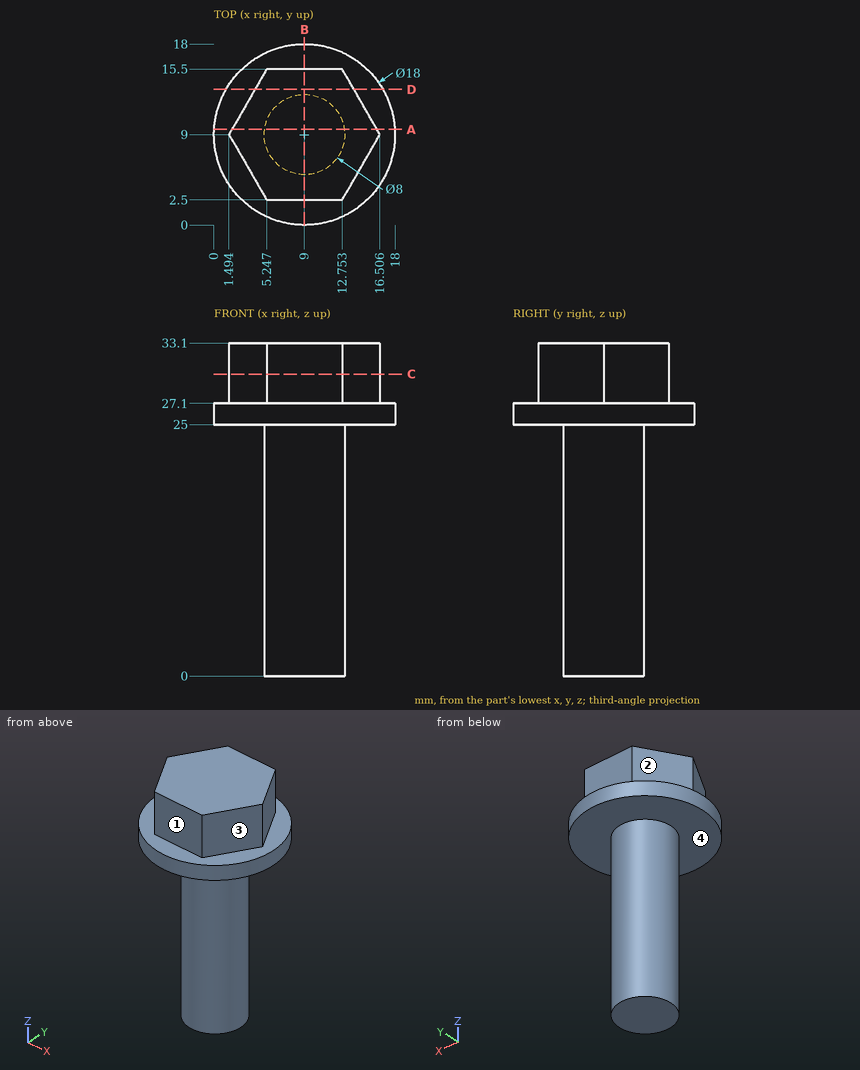
Geometry check sheet. Reference: drawing and pictorial views, mm from the part's lowest x, y, z. A direction names the side the tool comes from. Round coordinates to 2 decimals unless told otherwise and drop trailing zeros. Order: outer loops, then holes, each group sorted by start corner. A loop starts at its lowest first (then second) coordinate and runs counter-clockwise, first axis right, second up. Notation, with made-up numbers: M -37,-32 L -25,-32 A15 cw -25,-3 Z; hole C 22.5,54.25 d9. An arc over 180 degrees is marked long. Answer in a Markdown table with one row per item.
(1) Tool access check on the marked faces 1, 2, 3 and 4. Record the directions out of +Z, -Z, +X, -X, +Y, -Y that give a thin tool (end or side, any length) a straight path to the whole face; none if there is none.
Responses:
| item | result |
|---|---|
| face 1 | +Z, +X, -X, -Y |
| face 2 | +Z, -X, +Y |
| face 3 | +Z, +X, -Y |
| face 4 | -Z |
(2) Sectioned sample at A-A, the plane y = 9.5. Record the cut outline in (x, z).
Responses:
| item | result |
|---|---|
| outline | M 0.01,25 L 5.03,25 L 5.03,0 L 12.97,0 L 12.97,25 L 17.99,25 L 17.99,27.1 L 16.22,27.1 L 16.22,33.1 L 1.78,33.1 L 1.78,27.1 L 0.01,27.1 Z |
(3) Sectioned sample at D-D, the plane y = 13.5. Record the cut outline in (x, z) (1 decimal).
Responses:
| item | result |
|---|---|
| outline | M 1.2,25 L 16.8,25 L 16.8,27.1 L 13.9,27.1 L 13.9,33.1 L 4.1,33.1 L 4.1,27.1 L 1.2,27.1 Z |
(4) Sectioned sample at B-B, the plane x = 9. Record the cut outline in (y, z).
Responses:
| item | result |
|---|---|
| outline | M 0,25 L 5,25 L 5,0 L 13,0 L 13,25 L 18,25 L 18,27.1 L 15.5,27.1 L 15.5,33.1 L 2.5,33.1 L 2.5,27.1 L 0,27.1 Z |
(5) Sectioned sample at C-C, the plane z = 30. Record the cut outline in (x, y) (1 decimal), and give its area (3 significant figures).
Responses:
| item | result |
|---|---|
| outline | M 1.5,9 L 5.2,2.5 L 12.8,2.5 L 16.5,9 L 12.8,15.5 L 5.2,15.5 Z |
| area | 146 mm² |
(6) Go/stop test with flat-tipped pins: P1, Ø10, axis at x = 2, z = 6.5, coming from the -Y side (1 decimal); P2, Ø3, axis at x = 3, z = 25.5, coming from the -Y side (1 decimal); P3, Ø6.5, axis at x = 9, z = 31, coming from the -Y side. Record where each tip stops, or that it passes through.
Responses:
| item | result |
|---|---|
| P1 | stops at y = 5.5 |
| P2 | stops at y = 1.2 |
| P3 | stops at y = 2.5 |
(7) Scan lines: probe 1 along Z at (x, y) = (10, 17); probe 2 along Z at (x, y) = (6.25, 3); probe 3 along Y at (x, z) = (9, 12.5). Record each from-to range of solid material in increasing order. Write a range as from..to.
Responses:
| item | result |
|---|---|
| probe 1 | z = 25..27.1 |
| probe 2 | z = 25..33.1 |
| probe 3 | y = 5..13 |
